Verification items for the finished model (mm, model axes). A direction names the side the tool comes from. Round coordinates to 2 decimals unless told otherwise and drop trailing zeros. Order: outer loops, then holes, each group sorted by start corner. A loop starts at its lowest first (then second) coordinate and runs counter-clockwise, first axis right, second up. Notation, with made-up numbers: (78.25, 34) -> (121.25, 34) arc R25 cw to (121.25, 73) -> close; hole circle Ø11 at (67.5, 53.5). An arc over 180 degrees is marked (long way). Return JSON: item names as keys, results as strings. Group by question number.
Item 1: Scan lines: probe 1 along Y at (x, z) = (0, -811); probe 2 along Z at (x, y) = (-0.25, -0.25); probe 3 along X at (y, z) = (2.75, 334). Record each from-to range of solid material in increasing order. Write a range as from..to.
Item 2: Access from +Z, -Z, +X, -X, +Y, -Y to the whole of each face (thin tool, end or side, straight path). Record for faces 1 (the cylindrical face through (11.923, 3.755, 240.091)), 2 (the flat face through (3, 3, -823)), 3 (the cylindrical face through (5.77, 11.09, -686.11)).
Item 3: Sectioned sample at B-B on z = 243. Record the cut outline in (x, y).
Item 4: Depth check by flat-ended pin: pin 1 Ø2.5 at (x, z) = (-0.5, -772) entering from -Y; pin 2 Ø10 at (x, z) = (1, -44) entering from +Y; pin 3 Ø12 at (y, z) = (-7, -169.5) entering from -X. Enter the tip coordinate at first touch or a pass-through.
Item 5: Sectioned sample at A-A on z = -345. Record the cut outline in (x, y).
```python
from build123d import *

# Parameters (mm, degrees)
F0_R      = 12.5
F1_DEPTH  = 462
F2_R      = 12.5
F3_DEPTH  = 25
F5_DEPTH  = 553
F6_R      = 12.5
F7_DEPTH  = 270
F10_DEPTH = 2.5
F12_D     = 6.8
F12_DEPTH = 20
F12_TIP   = 2.0429261047


with BuildPart() as f1:
    # F0 (on Top) → F1 (new body)
    with BuildSketch(Plane.XY):
        Circle(F0_R)
    extrude(amount=F1_DEPTH)

    # F2 (on face) → F3 (join)
    with BuildSketch(Plane.XY.offset(462)):
        Circle(F2_R)
    extrude(amount=F3_DEPTH)

    # F4 (on face) → F5 (join)
    with BuildSketch(Plane(origin=(0, 0, 0), x_dir=(1, 0, 0), z_dir=(0, 0, -1))):
        Polygon((14.4297718574, 0.3391422642), (6.9211801124, 12.6661201315), (-7.508591745, 12.3269778673), (-14.4297718574, -0.3391422642), (-6.9211801124, -12.6661201315), (7.508591745, -12.3269778673), align=None)
    extrude(amount=F5_DEPTH)

    # F6 (on face) → F7 (join)
    with BuildSketch(Plane(origin=(0, 0, -553), x_dir=(1, 0, 0), z_dir=(0, 0, -1))):
        Circle(F6_R)
    extrude(amount=F7_DEPTH)

    # F9 (on offset) → F10 (cut)
    with BuildSketch(Plane.XZ.offset(12.5)):
        with BuildLine():
            ThreePointArc((-3.81, -797.19), (0, -801), (3.81, -797.19))
            Line((3.81, -797.19), (3.81, -704.81))
            ThreePointArc((3.81, -704.81), (0, -701), (-3.81, -704.81))
            Line((-3.81, -704.81), (-3.81, -797.19))
        make_face()
    extrude(amount=-F10_DEPTH, mode=Mode.SUBTRACT)

    # F12
    with Locations(Plane(origin=(0, 0, -823), x_dir=(1, 0, 0), z_dir=(0, 0, -1))):
        with Locations((0, 0)):
            Hole(F12_D / 2, depth=F12_DEPTH)
            with Locations((0, 0, -(F12_DEPTH + F12_TIP / 2))):  # 118° drill point
                Cone(0, F12_D / 2, F12_TIP, mode=Mode.SUBTRACT)


solid = f1.part
```
Recorded:
{
 "1": {"probe 1": "-12.5..-3.4, 3.4..12.5", "probe 2": "-801.17..487", "probe 3": "-12.19..12.19"},
 "2": {"face 1": "+Z", "face 2": "-Z, +X, -X, +Y, -Y", "face 3": "-Z"},
 "3": {"outline": "circle Ø25 at (0, 0)"},
 "4": {"pin 1": "y = -10", "pin 2": "y = 12.6", "pin 3": "x = -13.7"},
 "5": {"outline": "(-14.43, 0.34) -> (-7.51, -12.33) -> (6.92, -12.67) -> (14.43, -0.34) -> (7.51, 12.33) -> (-6.92, 12.67) -> close"}
}
